Work out the finished part from the listing and answer in its coordinate system (mm). Round coordinates to 2 decimals unless told otherwise and drop trailing zeros. Write each loop counter-clockwise with the first axis right and the second up, starting at its lowest first coordinate (ties: lowest second). Pieces come first, ordered by that corner, then holes.
from build123d import *

# Parameters (mm, degrees)
SKETCH1_R            = 0.5
BOSS_EXTRUDE1_DEPTH  = 0.1
SKETCH2_W            = 38.1
SKETCH2_H            = 7.62
BOSS_EXTRUDE2_DEPTH  = 1
LPATTERN2_COUNT      = 5
LPATTERN2_PITCH      = 7.62
LPATTERN2_COUNT_DIR2 = 3
LPATTERN2_PITCH_DIR2 = 2.54
SKETCH3_R            = 0.5
CUT_EXTRUDE1_DEPTH   = 38.386781086


with BuildPart() as part:
    # Sketch1 → Boss-Extrude1 (new body)
    with BuildSketch(Plane(origin=(0, 0, 0), x_dir=(1, 0, 0), z_dir=(0, 1, 0))):
        with BuildLine():
            Line((0, 0.75), (5.08, 0.75))
            ThreePointArc((5.08, 0.75), (5.83, 0), (5.08, -0.75))
            Line((5.08, -0.75), (0, -0.75))
            ThreePointArc((0, -0.75), (-0.75, 0), (0, 0.75))
        make_face()
        with Locations(Location((0, 0, 0), (0, 0, 270))):
            Circle(SKETCH1_R, mode=Mode.SUBTRACT)
        with Locations(Location((2.54, 0, 0), (0, 0, 270))):
            Circle(SKETCH1_R, mode=Mode.SUBTRACT)
        with Locations(Location((5.08, 0, 0), (0, 0, 270))):
            Circle(SKETCH1_R, mode=Mode.SUBTRACT)
    boss_extrude1 = extrude(amount=BOSS_EXTRUDE1_DEPTH)

    # Sketch2 → Boss-Extrude2 (add)
    with BuildSketch(Plane(origin=(0, 0, 0), x_dir=(1, 0, 0), z_dir=(0, 1, 0))):
        with Locations((17.78, 2.54)):
            Rectangle(SKETCH2_W, SKETCH2_H)
    extrude(amount=-BOSS_EXTRUDE2_DEPTH)

    # LPattern2: Boss-Extrude1 5 × 3
    with Locations(*[(i * LPATTERN2_PITCH, 0, -j * LPATTERN2_PITCH_DIR2) for i in range(LPATTERN2_COUNT) for j in range(LPATTERN2_COUNT_DIR2) if (i, j) != (0, 0)]):
        add(boss_extrude1)

    # Sketch3 → Cut-Extrude1 (cut, through all)
    with BuildSketch(Plane(origin=(0, 0, 0), x_dir=(1, 0, 0), z_dir=(0, 1, 0))):
        with Locations(Location((0, 0, 0), (0, 0, 270))):
            Circle(SKETCH3_R)
        with Locations(Location((2.54, 0, 0), (0, 0, 270))):
            Circle(SKETCH3_R)
        with Locations(Location((5.08, 0, 0), (0, 0, 270))):
            Circle(SKETCH3_R)
        with Locations(Location((7.62, 0, 0), (0, 0, 270))):
            Circle(SKETCH3_R)
        with Locations(Location((10.16, 0, 0), (0, 0, 270))):
            Circle(SKETCH3_R)
        with Locations(Location((12.7, 0, 0), (0, 0, 270))):
            Circle(SKETCH3_R)
        with Locations(Location((15.24, 0, 0), (0, 0, 270))):
            Circle(SKETCH3_R)
        with Locations(Location((17.78, 0, 0), (0, 0, 270))):
            Circle(SKETCH3_R)
        with Locations(Location((20.32, 0, 0), (0, 0, 270))):
            Circle(SKETCH3_R)
        with Locations(Location((22.86, 0, 0), (0, 0, 270))):
            Circle(SKETCH3_R)
        with Locations(Location((25.4, 0, 0), (0, 0, 270))):
            Circle(SKETCH3_R)
        with Locations(Location((27.94, 0, 0), (0, 0, 270))):
            Circle(SKETCH3_R)
        with Locations(Location((30.48, 0, 0), (0, 0, 270))):
            Circle(SKETCH3_R)
        with Locations(Location((33.02, 0, 0), (0, 0, 270))):
            Circle(SKETCH3_R)
        with Locations(Location((35.56, 0, 0), (0, 0, 270))):
            Circle(SKETCH3_R)
        with Locations(Location((0, 2.54, 0), (0, 0, 270))):
            Circle(SKETCH3_R)
        with Locations(Location((2.54, 2.54, 0), (0, 0, 270))):
            Circle(SKETCH3_R)
        with Locations(Location((5.08, 2.54, 0), (0, 0, 270))):
            Circle(SKETCH3_R)
        with Locations(Location((7.62, 2.54, 0), (0, 0, 270))):
            Circle(SKETCH3_R)
        with Locations(Location((10.16, 2.54, 0), (0, 0, 270))):
            Circle(SKETCH3_R)
        with Locations(Location((12.7, 2.54, 0), (0, 0, 270))):
            Circle(SKETCH3_R)
        with Locations(Location((15.24, 2.54, 0), (0, 0, 270))):
            Circle(SKETCH3_R)
        with Locations(Location((17.78, 2.54, 0), (0, 0, 270))):
            Circle(SKETCH3_R)
        with Locations(Location((20.32, 2.54, 0), (0, 0, 270))):
            Circle(SKETCH3_R)
        with Locations(Location((22.86, 2.54, 0), (0, 0, 270))):
            Circle(SKETCH3_R)
        with Locations(Location((25.4, 2.54, 0), (0, 0, 270))):
            Circle(SKETCH3_R)
        with Locations(Location((27.94, 2.54, 0), (0, 0, 270))):
            Circle(SKETCH3_R)
        with Locations(Location((30.48, 2.54, 0), (0, 0, 270))):
            Circle(SKETCH3_R)
        with Locations(Location((33.02, 2.54, 0), (0, 0, 270))):
            Circle(SKETCH3_R)
        with Locations(Location((35.56, 2.54, 0), (0, 0, 270))):
            Circle(SKETCH3_R)
        with Locations(Location((0, 5.08, 0), (0, 0, 270))):
            Circle(SKETCH3_R)
        with Locations(Location((2.54, 5.08, 0), (0, 0, 270))):
            Circle(SKETCH3_R)
        with Locations(Location((5.08, 5.08, 0), (0, 0, 270))):
            Circle(SKETCH3_R)
        with Locations(Location((7.62, 5.08, 0), (0, 0, 270))):
            Circle(SKETCH3_R)
        with Locations(Location((10.16, 5.08, 0), (0, 0, 270))):
            Circle(SKETCH3_R)
        with Locations(Location((12.7, 5.08, 0), (0, 0, 270))):
            Circle(SKETCH3_R)
        with Locations(Location((15.24, 5.08, 0), (0, 0, 270))):
            Circle(SKETCH3_R)
        with Locations(Location((17.78, 5.08, 0), (0, 0, 270))):
            Circle(SKETCH3_R)
        with Locations(Location((20.32, 5.08, 0), (0, 0, 270))):
            Circle(SKETCH3_R)
        with Locations(Location((22.86, 5.08, 0), (0, 0, 270))):
            Circle(SKETCH3_R)
        with Locations(Location((25.4, 5.08, 0), (0, 0, 270))):
            Circle(SKETCH3_R)
        with Locations(Location((27.94, 5.08, 0), (0, 0, 270))):
            Circle(SKETCH3_R)
        with Locations(Location((30.48, 5.08, 0), (0, 0, 270))):
            Circle(SKETCH3_R)
        with Locations(Location((33.02, 5.08, 0), (0, 0, 270))):
            Circle(SKETCH3_R)
        with Locations(Location((35.56, 5.08, 0), (0, 0, 270))):
            Circle(SKETCH3_R)
    extrude(amount=-CUT_EXTRUDE1_DEPTH, mode=Mode.SUBTRACT)


solid = part.part
Q1. Find section C-C (x = 27). Determine the outline of the cut face in (y, z), plus the area to 3 significant figures.
Q2. Find section A-A (x = 10.16). Determine the outline of the cut face in (y, z), plus the area to 3 significant figures.
Q3. Find section B-B (z = -2.54). Count the separate pieces of the cut face and the enclosed holes in it, plus the area to 3 significant figures.
Q4. Find the intervals of material crossed by L1, parallel to Z at x = 28, y = -0.25; L2, parallel to Z at x = 8, y = -0.8; L3, parallel to Y at x = 29.5, z = -1.25, in increasing order.
Report:
1. outline: (-1, -6.35) - (0, -6.35) - (0, -5.83) - (0.1, -5.83) - (0.1, -4.33) - (0, -4.33) - (0, -3.29) - (0.1, -3.29) - (0.1, -1.79) - (0, -1.79) - (0, -0.75) - (0.1, -0.75) - (0.1, 0.75) - (0, 0.75) - (0, 1.27) - (-1, 1.27) - close
1. area: 8.07 mm2
2. outline: (-1, -6.35) - (0, -6.35) - (0, -5.83) - (0.1, -5.83) - (0.1, -5.58) - (-1, -5.58) - close; (-1, -4.58) - (0.1, -4.58) - (0.1, -4.33) - (0, -4.33) - (0, -3.29) - (0.1, -3.29) - (0.1, -3.04) - (-1, -3.04) - close; (-1, -2.04) - (0.1, -2.04) - (0.1, -1.79) - (0, -1.79) - (0, -0.75) - (0.1, -0.75) - (0.1, -0.5) - (-1, -0.5) - close; (-1, 0.5) - (0.1, 0.5) - (0.1, 0.75) - (0, 0.75) - (0, 1.27) - (-1, 1.27) - close
2. area: 4.77 mm2
3. separate pieces: 16
3. enclosed holes: 0
3. area: 24.9 mm2
4. L1: z = -6.35 to -5.58, -4.58 to -3.04, -2.04 to -0.5, 0.5 to 1.27
4. L2: z = -6.35 to -5.4, -4.76 to -2.86, -2.22 to -0.32, 0.32 to 1.27
4. L3: y = -1 to 0
